from build123d import *

# Parameters (mm, degrees)
BOSS_EXTRUDE1_DEPTH = 5


with BuildPart() as part:
    # Sketch1 → Boss-Extrude1 (new body)
    with BuildSketch(Plane(origin=(0, 0, 0), x_dir=(1, 0, 0), z_dir=(0, 1, 0))):
        with BuildLine():
            Line((7, 36.2), (10, 36.2))
            ThreePointArc((10, 36.2), (11.414213562, 35.614213562), (12, 34.2))
            Line((12, 34.2), (12, 24.5))
            ThreePointArc((12, 24.5), (11.414213562, 23.085786438), (10, 22.5))
            Line((10, 22.5), (7, 22.5))
            ThreePointArc((7, 22.5), (5.585786438, 21.914213562), (5, 20.5))
            Line((5, 20.5), (5, 2))
            ThreePointArc((5, 2), (4.414213562, 0.585786438), (3, 0))
            Line((3, 0), (0, 0))
            Line((0, 0), (0, 27.5))
            Line((0, 27.5), (7, 27.5))
            Line((7, 27.5), (7, 36.2))
        make_face()
    extrude(amount=BOSS_EXTRUDE1_DEPTH)


solid = part.part
For this review, take the finished solid that the model builds, in its own axes (mm). A direction names the side the tool comes from. Coordinates: 2 decimals unless noted, no trailing zeros. Write each loop counter-clockwise with the first axis right and the second up, starting at its lowest first coordinate (ties: lowest second). Pieces come first, ordered by that corner, then holes. Notation, with made-up numbers: (84.25, -39.5) -> (125.25, -39.5) arc R13 cw to (125.25, -25.5) -> close; hole circle Ø11 at (-29, 56). An arc over 180 degrees is marked (long way). Write each question's results on one line, items separated by ' | '. Start each with the question number.
1) Insertion check: pin 1 (2 mm diameter, centred on y = 4.5, z = -13.5, fed in from +X). The pin has a flat end and moves straight along its axis. Give the tip position at first contact, or say it passes through.
2) Wall thickness on L1, parallel to Z at x = 9.25, y = 1.75; L2, parallel to Z at x = 2, y = 2; L3, parallel to X at y = 0.4, z = -11.5: over which ranges is each line inside the solid? List them lowest first. Write a range as [from, to].
3) For faces 1 (the face through (9, 2, -22.5)), 2 (the face through (7, 2, -32)), 3 (the face through (12, 2, -29)), list the 3-axis set-ups (+Z, -Z, +X, -X, +Y, -Y) from which the entire face can be reached by the end or side of a thin tool; tool diameter is ignored.
4) Consider section B-B (z = -2.5). Write out the cut boundary in (x, y), plus the area to 3 significant figures.
5) Consider section A-A (y = 0.7). Write out the cut boundary in (x, z).
6) Consider section C-C (x = 8.25). Write out the cut boundary in (y, z), plus the area to 3 significant figures.
Geometry says:
1) pin 1: x = 5
2) L1: [-36.2, -22.5] | L2: [-27.5, 0] | L3: [0, 5]
3) face 1: +Z, +X, +Y, -Y | face 2: -Z, -X, +Y, -Y | face 3: +Z, -Z, +X, +Y, -Y
4) outline: (0, 0) -> (5, 0) -> (5, 5) -> (0, 5) -> close | area: 25.0 mm^2
5) outline: (0, -27.5) -> (7, -27.5) -> (7, -36.2) -> (10, -36.2) arc R2 ccw to (12, -34.2) -> (12, -24.5) arc R2 ccw to (10, -22.5) -> (7, -22.5) arc R2 cw to (5, -20.5) -> (5, -2) arc R2 ccw to (3, 0) -> (0, 0) -> close
6) outline: (0, -36.2) -> (5, -36.2) -> (5, -22.5) -> (0, -22.5) -> close | area: 68.5 mm^2
